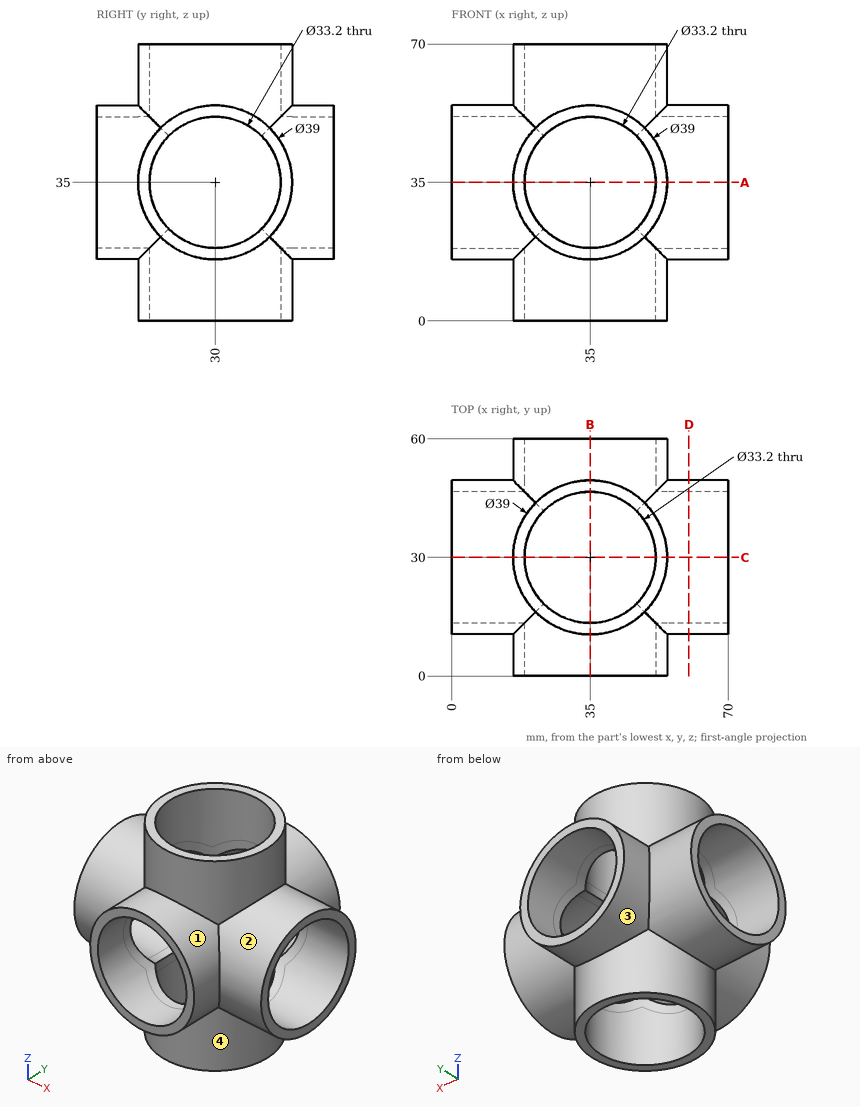
Answer from the drawing. Dimensions are ordinates in mm from the lowest x, y and z of the part. A direction names the side the tool comes from. Round coordinates to 2 decimals unless told otherwise and drop trailing zeros. Write each loop counter-clockwise with the first axis right and the second up, starting at its lowest first coordinate (ties: lowest second). Pieces come first, ordered by that corner, then holes.
1. The part is cut by section D-D, the plane x = 60. Determine the outline of the cut face in (y, z), then the cut area to 3 significant figures.
2. The part is cut by section C-C, the plane y = 30. Determine the outline of the cut face in (x, z), then the cut area to 3 significant figures.
3. The part is cut by section A-A, the plane z = 35. Determine the outline of the cut face in (x, y).
4. Which of the six approach directions +Z, -Z, +X, -X, +Y, -Y give full straight-line access (tool end or side, diameter ignored) to the marked faces 1, 2, 3 and 4?
5. Straight lines are drawn through the part: L1, parallel to Y at x = 56.25, z = 35; L2, parallel to Z at x = 55.5, y = 27.5; L3, parallel to X at y = 29, z = 54. For each, find the intervals that lie inside material, in ascending order.
6. The part is cut by section B-B, the plane x = 35. Determine the outline of the cut face in (y, z).
7. Given pin 1 Ø4 at (y, z) = (13, 12) entering from -X; pin 2 Ø20 at (x, z) = (35, 35) entering from -Y; pin 3 Ø10 at (x, y) = (13, 10.5) entering from +Z; pin 4 Ø12 at (x, z) = (9, 51.5) entering from -Y, each flat-ended and moving along its own axis, determine where each tip first touches the part or whether it passes through.
Values:
1. outline: circle Ø39 at (30, 35); hole circle Ø33.2 at (30, 35)
1. area: 329 mm2
2. outline: (0, 15.5) - (15.5, 15.5) - (15.5, 0) - (18.4, 0) - (18.4, 18.4) - (0, 18.4) - close; (0, 51.6) - (18.4, 51.6) - (18.4, 70) - (15.5, 70) - (15.5, 54.5) - (0, 54.5) - close; (51.6, 0) - (54.5, 0) - (54.5, 15.5) - (70, 15.5) - (70, 18.4) - (51.6, 18.4) - close; (51.6, 51.6) - (70, 51.6) - (70, 54.5) - (54.5, 54.5) - (54.5, 70) - (51.6, 70) - close
2. area: 393 mm2
3. outline: (0, 10.5) - (15.5, 10.5) - (15.5, 0) - (18.4, 0) - (18.4, 13.4) - (0, 13.4) - close; (0, 46.6) - (18.4, 46.6) - (18.4, 60) - (15.5, 60) - (15.5, 49.5) - (0, 49.5) - close; (51.6, 0) - (54.5, 0) - (54.5, 10.5) - (70, 10.5) - (70, 13.4) - (51.6, 13.4) - close; (51.6, 46.6) - (70, 46.6) - (70, 49.5) - (54.5, 49.5) - (54.5, 60) - (51.6, 60) - close
4. face 1: -Y
4. face 2: +X
4. face 3: +Y
4. face 4: -Z
5. L1: y = 10.5 to 13.4, 46.6 to 49.5
5. L2: z = 15.66 to 18.59, 51.41 to 54.34
5. L3: x = 0 to 18.43, 51.57 to 70
6. outline: (0, 15.5) - (10.5, 15.5) - (10.5, 0) - (13.4, 0) - (13.4, 18.4) - (0, 18.4) - close; (0, 51.6) - (13.4, 51.6) - (13.4, 70) - (10.5, 70) - (10.5, 54.5) - (0, 54.5) - close; (46.6, 0) - (49.5, 0) - (49.5, 15.5) - (60, 15.5) - (60, 18.4) - (46.6, 18.4) - close; (46.6, 51.6) - (60, 51.6) - (60, 54.5) - (49.5, 54.5) - (49.5, 70) - (46.6, 70) - close
7. pin 1: stops at x = 22.54
7. pin 2: passes through
7. pin 3: stops at z = 48.04
7. pin 4: stops at y = 13.57
